Check sheet for the modelled part. Datum: model origin and axes. Units: mm. A direction names the side the tool comes from. Give positions to 0.01 mm unless a question says otherwise; leave off trailing zeros. Order: outer loops, then holes, each group sorted by start corner. A loop starts at its lowest first (then second) coordinate and runs counter-clockwise, first axis right, second up.
from build123d import *

# Parameters (mm, degrees)
SKETCH_2_W      = 160
SKETCH_2_H      = 160
EXTRUDE_1_DEPTH = 10
SKETCH_4_R      = 2.5
EXTRUDE_2_DEPTH = 85


with BuildPart() as part:
    # 草图2 → 凸台-拉伸1 (new body)
    with BuildSketch(Plane.XY):
        Rectangle(SKETCH_2_W, SKETCH_2_H)
    extrude(amount=EXTRUDE_1_DEPTH)

    # 草图4 → 凸台-拉伸2 (add, symmetric)
    with BuildSketch(Plane(origin=(0, 0, 0), x_dir=(1, 0, 0), z_dir=(0, 1, 0))):
        with Locations(Location((-65, -5, 0), (0, 0, 180))):
            Circle(SKETCH_4_R)
        with Locations(Location((65, -5, 0), (0, 0, 90))):
            Circle(SKETCH_4_R)
    extrude(amount=EXTRUDE_2_DEPTH, both=True)


solid = part.part
1) Draft check along X on faces 1 (the face through (-65, -85, 5)), 2 (the face through (-80, -1, 5)), 3 (the face through (67.22, 82.54, 3.85)), 4 (the face through (67.22, -82.46, 3.85)). Enter one of: +X half, -X half, draft (parallel to the pull), parting line (faces both ways), or undercut.
Recorded:
face 1: draft
face 2: -X half
face 3: undercut
face 4: undercut
2) Depth check by flat-ended pin: pin 1 Ø1.5 at (x, z) = (-16.5, 6) entering from +Y; pin 2 Ø5 at (x, z) = (-20.5, 7.5) entering from -Y. Enter the tip coordinate at first touch or a pass-through.
Recorded:
pin 1: stops at y = 80
pin 2: stops at y = -80
3) Set-up check for faces 5 (the face through (-67.385, -82.465, 5.751)), 6 (the face through (80, -1, 5)), 7 (the face through (-67.385, 82.465, 5.751)): record each of +Z, -Z, +X, -X, +Y, -Y from which the full face is reachable in a straight line by a thin tool's end or side.
Recorded:
face 5: -Y
face 6: +Z, -Z, +X, +Y, -Y
face 7: +Y
4) Section check B-B, the plane x = 65. Record the cut outline in (y, z).
Recorded:
outline: (-85, 2.5) - (-80, 2.5) - (-80, 0) - (80, 0) - (80, 2.5) - (85, 2.5) - (85, 7.5) - (80, 7.5) - (80, 10) - (-80, 10) - (-80, 7.5) - (-85, 7.5) - close
5) Section check A-A, the plane z = 5. Record the cut outline in (x, y).
Recorded:
outline: (-80, -80) - (-67.5, -80) - (-67.5, -85) - (-62.5, -85) - (-62.5, -80) - (62.5, -80) - (62.5, -85) - (67.5, -85) - (67.5, -80) - (80, -80) - (80, 80) - (67.5, 80) - (67.5, 85) - (62.5, 85) - (62.5, 80) - (-62.5, 80) - (-62.5, 85) - (-67.5, 85) - (-67.5, 80) - (-80, 80) - close
6) Section check C-C, the plane x = 5.5. Record the cut outline in (y, z).
Recorded:
outline: (-80, 0) - (80, 0) - (80, 10) - (-80, 10) - close
7) Material ranges on L1, parallel to Y at x = 55, z = 4, recorded low to high.
Recorded:
L1: y = -80 to 80
